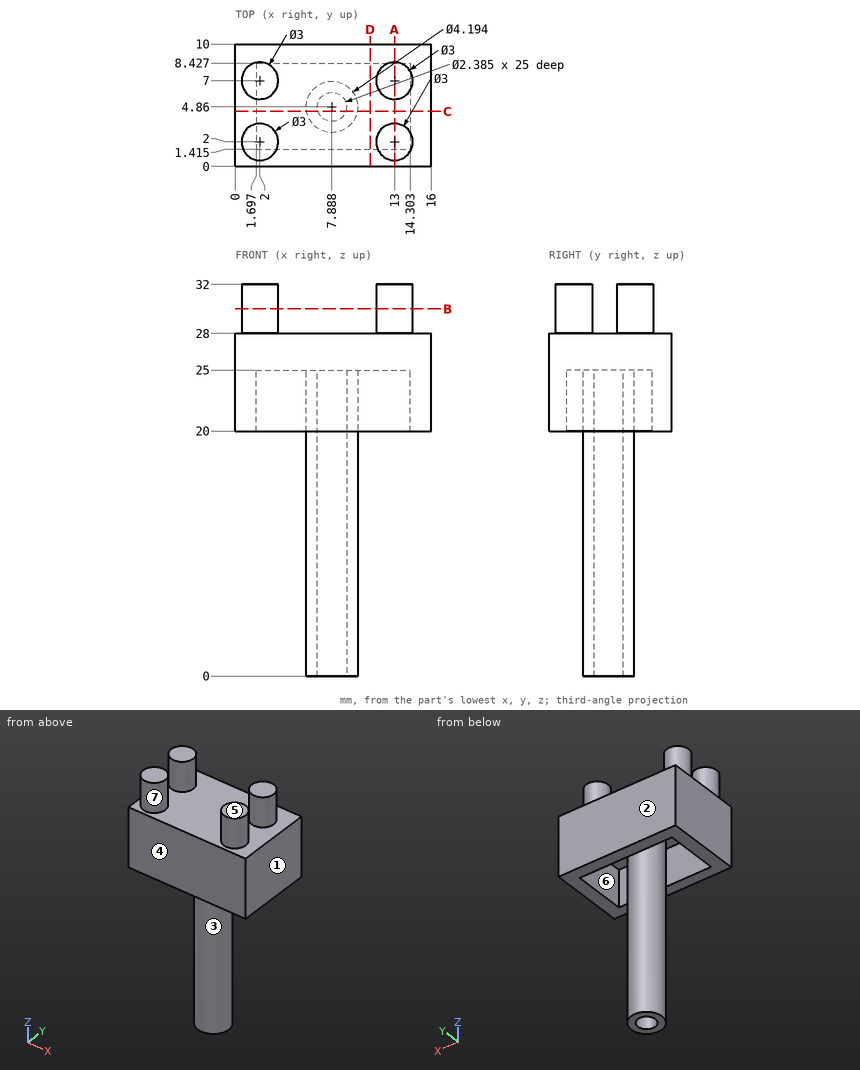
Check sheet for the drawn part. Datum: minimum x, y, z corner. Units: mm. A direction names the side the tool comes from. Round coordinates to 2 decimals unless told otherwise and drop trailing zeros. Order: outer loops, then holes, each group sorted by start corner. A loop starts at its lowest first (then second) coordinate and runs counter-clockwise, first axis right, second up.
1. Section check C-C on y = 4.5. Record the cut outline in (x, z) (1 decimal).
Final values:
outline: (0, 20) - (1.7, 20) - (1.7, 25) - (5.8, 25) - (5.8, 0) - (6.8, 0) - (6.8, 25) - (9, 25) - (9, 0) - (10, 0) - (10, 25) - (14.3, 25) - (14.3, 20) - (16, 20) - (16, 28) - (0, 28) - close
2. Release check for a two-part mould opening along Y. For the marked faces 1, 2, 3 and 4 record: +Y half, -Y half, draft (parallel to the pull), parting line (faces both ways), or undercut.
Final values:
face 1: draft
face 2: +Y half
face 3: undercut
face 4: -Y half
3. Access from +Z, -Z, +X, -X, +Y, -Y to the whole of each face (thin tool, end or side, straight path). Record for the marked faces 5, 6 and 7.
Final values:
face 5: +Z, +X, -X, +Y, -Y
face 6: -Z
face 7: +Z
4. Thickness scan on L1, parallel to Y at x = 8, z = 13 (1 decimal); L2, parallel to X at y = 4.75, z = 23.5 (1 decimal); L3, parallel to X at y = 7.75, z = 20.5. Record the ranges inside material, lowest first.
Final values:
L1: y = 2.8 to 3.7, 6 to 7
L2: x = 0 to 1.7, 5.8 to 6.7, 9.1 to 10, 14.3 to 16
L3: x = 0 to 1.7, 14.3 to 16
5. Go/stop test with flat-tipped pins: P1, Ø2, axis at x = 7.89, y = 4.86, coming from the +Z side; P2, Ø5, axis at x = 11, z = 9, coming from the -Y side; P3, Ø1.5, axis at y = 5, z = 14, coming from the -X side. Record where each tip stops, or that it passes through.
Final values:
P1: stops at z = 28
P2: stops at y = 2.85
P3: stops at x = 5.79
6. Section check B-B on z = 30. Record the cut outline in (x, y).
Final values:
outline: circle Ø3 at (2, 2); circle Ø3 at (2, 7); circle Ø3 at (13, 2); circle Ø3 at (13, 7)
7. Section check D-D on x = 11. Record the cut outline in (y, z) (1 decimal).
Final values:
outline: (0, 20) - (1.4, 20) - (1.4, 25) - (8.4, 25) - (8.4, 20) - (10, 20) - (10, 28) - (0, 28) - close
8. Section check A-A on x = 13. Record the cut outline in (y, z) (1 decimal).
Final values:
outline: (0, 20) - (1.4, 20) - (1.4, 25) - (8.4, 25) - (8.4, 20) - (10, 20) - (10, 28) - (8.5, 28) - (8.5, 32) - (5.5, 32) - (5.5, 28) - (3.5, 28) - (3.5, 32) - (0.5, 32) - (0.5, 28) - (0, 28) - close
